```python
from build123d import *
from build123d.topology import SkipClean

# Parameters (mm, degrees)
SKETCH_1_R               = 30
EXTRUDE_1_DEPTH          = 8
CUT_EXTRUDE_5_DEPTH      = 905.685953271
CUT_EXTRUDE_5_DEPTH_BACK = 905.685953271
SKETCH_8_R               = 2.25
SKETCH_9_R               = 4
CUT_EXTRUDE_6_DEPTH      = 4.4
FILLET_1_R               = 100
CUT_EXTRUDE_7_DEPTH      = 83
CUT_EXTRUDE_8_DEPTH      = 83
FILLET_3_R               = 100
FILLET_4_R               = 10
SKETCH_14_R              = 4.25
CUT_EXTRUDE_9_DEPTH      = 83
EXTRUDE_2_DEPTH          = 5
CUT_EXTRUDE_10_DEPTH     = 69
FILLET_5_R               = 10
CHAMFER_1_SIZE           = 5
CHAMFER_2_SIZE           = 5


with BuildPart() as part:
    # 草图1 → 凸台-拉伸1 (new body)
    with BuildSketch(Plane.XY):
        Polygon((0, 250), (769.420884294, 0), (0, 0), (-100, 0), (-869.420884294, 0), (-100, 250), align=None)
        with Locations((100, 100)):
            Circle(SKETCH_1_R, mode=Mode.SUBTRACT)
        with Locations(Location((-200, 100, 0), (0, 0, 180))):
            Circle(SKETCH_1_R, mode=Mode.SUBTRACT)
    extrude(amount=EXTRUDE_1_DEPTH)

    # 草图8 → 切除-拉伸5 (cut, two sides: drawn at the far end of the back side and taken through both)
    with BuildSketch(Plane.XY.offset(8).offset(-CUT_EXTRUDE_5_DEPTH_BACK)):
        with Locations((100, 141.5)):
            Circle(SKETCH_8_R)
        with Locations((129.344931419, 129.344931419)):
            Circle(SKETCH_8_R)
        with Locations((141.5, 100)):
            Circle(SKETCH_8_R)
        with Locations((129.344931419, 70.655068581)):
            Circle(SKETCH_8_R)
        with Locations((100, 58.5)):
            Circle(SKETCH_8_R)
        with Locations((70.655068581, 70.655068581)):
            Circle(SKETCH_8_R)
        with Locations((58.5, 100)):
            Circle(SKETCH_8_R)
        with Locations((70.655068581, 129.344931419)):
            Circle(SKETCH_8_R)
        with Locations(Location((-170.655068581, 129.344931419, 0), (0, 0, 180))):
            Circle(SKETCH_8_R)
        with Locations(Location((-158.5, 100, 0), (0, 0, 180))):
            Circle(SKETCH_8_R)
        with Locations(Location((-170.655068581, 70.655068581, 0), (0, 0, 180))):
            Circle(SKETCH_8_R)
        with Locations(Location((-200, 58.5, 0), (0, 0, 180))):
            Circle(SKETCH_8_R)
        with Locations(Location((-229.344931419, 70.655068581, 0), (0, 0, 180))):
            Circle(SKETCH_8_R)
        with Locations(Location((-241.5, 100, 0), (0, 0, 180))):
            Circle(SKETCH_8_R)
        with Locations(Location((-229.344931419, 129.344931419, 0), (0, 0, 180))):
            Circle(SKETCH_8_R)
        with Locations(Location((-200, 141.5, 0), (0, 0, 180))):
            Circle(SKETCH_8_R)
    extrude(amount=CUT_EXTRUDE_5_DEPTH + CUT_EXTRUDE_5_DEPTH_BACK, mode=Mode.SUBTRACT)

    # 草图9 → 切除-拉伸6 (cut)
    with BuildSketch(Plane.XY.offset(8)):
        with Locations((-200, 141.5)):
            Circle(SKETCH_9_R)
        with Locations((-170.655068581, 129.344931419)):
            Circle(SKETCH_9_R)
        with Locations((-158.5, 100)):
            Circle(SKETCH_9_R)
        with Locations((-170.655068581, 70.655068581)):
            Circle(SKETCH_9_R)
        with Locations((-200, 58.5)):
            Circle(SKETCH_9_R)
        with Locations((-229.344931419, 70.655068581)):
            Circle(SKETCH_9_R)
        with Locations((-241.5, 100)):
            Circle(SKETCH_9_R)
        with Locations((-229.344931419, 129.344931419)):
            Circle(SKETCH_9_R)
        with Locations(Location((129.344931419, 129.344931419, 0), (0, 0, 180))):
            Circle(SKETCH_9_R)
        with Locations(Location((141.5, 100, 0), (0, 0, 180))):
            Circle(SKETCH_9_R)
        with Locations(Location((129.344931419, 70.655068581, 0), (0, 0, 180))):
            Circle(SKETCH_9_R)
        with Locations(Location((100, 58.5, 0), (0, 0, 180))):
            Circle(SKETCH_9_R)
        with Locations(Location((70.655068581, 70.655068581, 0), (0, 0, 180))):
            Circle(SKETCH_9_R)
        with Locations(Location((58.5, 100, 0), (0, 0, 180))):
            Circle(SKETCH_9_R)
        with Locations(Location((70.655068581, 129.344931419, 0), (0, 0, 180))):
            Circle(SKETCH_9_R)
        with Locations(Location((100, 141.5, 0), (0, 0, 180))):
            Circle(SKETCH_9_R)
    extrude(amount=-CUT_EXTRUDE_6_DEPTH, mode=Mode.SUBTRACT)

    # 圆角1
    fillet_1_edges = [part.edges().sort_by_distance(p)[0] for p in [
        (-869.420884294, 0, 4),
        (769.420884294, 0, 4),
    ]]
    fillet(fillet_1_edges, radius=FILLET_1_R)

    # 草图12 → 切除-拉伸7 (cut)
    with BuildSketch(Plane(origin=(0, 0, 0), x_dir=(-1, 0, 0), z_dir=(0, 0, -1))):
        with BuildLine():
            Line((-20, 40), (120, 40))
            ThreePointArc((120, 40), (155.27864045, 10.5572809), (200, 0))
            Line((200, 0), (-100, 0))
            ThreePointArc((-100, 0), (-55.27864045, 10.5572809), (-20, 40))
        make_face()
    extrude(amount=-CUT_EXTRUDE_7_DEPTH, mode=Mode.SUBTRACT)

    # 草图13 → 切除-拉伸8 (cut)
    with BuildSketch(Plane.XY.offset(8)):
        with BuildLine():
            Line((-238.045732826, 0), (-200, 0))
            ThreePointArc((-200, 0), (-295.54722537, 70.491904093), (-256.388333797, 182.585445519))
            Line((-256.388333797, 182.585445519), (-210, 214.258833414))
            Line((-210, 214.258833414), (-268.947432264, 195.10565163))
            ThreePointArc((-268.947432264, 195.10565163), (-336.814566886, 84.356553496), (-238.045732826, 0))
        make_face()
        with BuildLine():
            Line((110, 214.258833414), (168.947432264, 195.10565163))
            ThreePointArc((168.947432264, 195.10565163), (236.814566886, 84.356553496), (138.045732826, 0))
            Line((138.045732826, 0), (100, 0))
            ThreePointArc((100, 0), (195.54722537, 70.491904093), (156.388333797, 182.585445519))
            Line((156.388333797, 182.585445519), (110, 214.258833414))
        make_face()
    extrude(amount=-CUT_EXTRUDE_8_DEPTH, mode=Mode.SUBTRACT)

    # 圆角3
    fillet_3_edges = [part.edges().sort_by_distance(p)[0] for p in [
        (-100, 250, 4),
        (0, 250, 4),
        (-210, 214.258833414, 4),
        (110, 214.258833414, 4),
    ]]
    fillet(fillet_3_edges, radius=FILLET_3_R)

    # 圆角4
    fillet_4_edges = [part.edges().sort_by_distance(p)[0] for p in [
        (20, 40, 4),
        (-120, 40, 4),
    ]]
    fillet(fillet_4_edges, radius=FILLET_4_R)

    # 草图14 → 切除-拉伸9 (cut)
    with BuildSketch(Plane.XY.offset(8)):
        with Locations((-35, 65)):
            Circle(SKETCH_14_R)
        with Locations((-35, 105)):
            Circle(SKETCH_14_R)
        with Locations((-35, 175)):
            Circle(SKETCH_14_R)
        with Locations((-35, 215)):
            Circle(SKETCH_14_R)
        with Locations(Location((-65, 215, 0), (0, 0, 180))):
            Circle(SKETCH_14_R)
        with Locations(Location((-65, 175, 0), (0, 0, 180))):
            Circle(SKETCH_14_R)
        with Locations(Location((-65, 105, 0), (0, 0, 180))):
            Circle(SKETCH_14_R)
        with Locations(Location((-65, 65, 0), (0, 0, 180))):
            Circle(SKETCH_14_R)
    extrude(amount=-CUT_EXTRUDE_9_DEPTH, mode=Mode.SUBTRACT)

    # 草图15 → 凸台-拉伸2 (add)
    with SkipClean():  # the faces are left unmerged after this step: merging them gives an invalid solid
        with BuildSketch(Plane(origin=(0, 0, 0), x_dir=(-1, 0, 0), z_dir=(0, 0, -1))):
            with BuildLine():
                Line((-15.063255405, 245.10565163), (-96.358782137, 218.691133779))
                ThreePointArc((-96.358782137, 218.691133779), (-109.548764066, 213.340279426), (-121.845416496, 206.170927668))
                Line((-121.845416496, 206.170927668), (-156.388333797, 182.585445519))
                ThreePointArc((-156.388333797, 182.585445519), (-173.843422805, 32.567449192), (-22.861078416, 36.363636364))
                ThreePointArc((-22.861078416, 36.363636364), (-19.411200585, 39.045340337), (-15.147186258, 40))
                Line((-15.147186258, 40), (115.147186258, 40))
                ThreePointArc((115.147186258, 40), (119.411200585, 39.045340337), (122.861078416, 36.363636364))
                ThreePointArc((122.861078416, 36.363636364), (273.843422805, 32.567449192), (256.388333797, 182.585445519))
                Line((256.388333797, 182.585445519), (221.845416496, 206.170927668))
                ThreePointArc((221.845416496, 206.170927668), (209.548764066, 213.340279426), (196.358782137, 218.691133779))
                Line((196.358782137, 218.691133779), (115.063255405, 245.10565163))
                ThreePointArc((115.063255405, 245.10565163), (99.805002472, 248.76883406), (84.161555968, 250))
                Line((84.161555968, 250), (15.838444032, 250))
                ThreePointArc((15.838444032, 250), (0.194997528, 248.76883406), (-15.063255405, 245.10565163))
            make_face()
            with BuildLine():
                Line((55, 50), (128.192966918, 50))
                ThreePointArc((128.192966918, 50), (262.154722909, 38.412335488), (249.339792072, 172.262264829))
                Line((249.339792072, 172.262264829), (197.086815625, 207.939959117))
                Line((197.086815625, 207.939959117), (98.416155597, 240))
                Line((98.416155597, 240), (55, 240))
                Line((55, 240), (55, 50))
            make_face(mode=Mode.SUBTRACT)
            with BuildLine():
                Line((45, 240), (45, 50))
                Line((45, 50), (-28.192966918, 50))
                ThreePointArc((-28.192966918, 50), (-162.154722909, 38.412335488), (-149.339792072, 172.262264829))
                Line((-149.339792072, 172.262264829), (-97.086815625, 207.939959117))
                Line((-97.086815625, 207.939959117), (1.583844403, 240))
                Line((1.583844403, 240), (45, 240))
            make_face(mode=Mode.SUBTRACT)
        extrude(amount=EXTRUDE_2_DEPTH)

    # 草图16 → 切除-拉伸10 (cut)
    with SkipClean():  # the faces are left unmerged after this step: merging them gives an invalid solid
        with BuildSketch(Plane(origin=(0, 0, 0), x_dir=(-1, 0, 0), z_dir=(0, 0, -1))):
            Polygon((80, 230), (80, 130), (166.602540378, 180), align=None)
            Polygon((-66.602540378, 180), (20, 230), (20, 130), align=None)
        extrude(amount=-CUT_EXTRUDE_10_DEPTH, mode=Mode.SUBTRACT)

    # 圆角5
    fillet_5_edges = [part.edges().sort_by_distance(p)[0] for p in [
        (-197.086815625, 207.939959117, -2.5),
        (-98.416155597, 240, -2.5),
        (-55, 240, -2.5),
        (-55, 50, -2.5),
        (-128.192966918, 50, -2.5),
        (28.192966918, 50, -2.5),
        (-45, 50, -2.5),
        (-45, 240, -2.5),
        (-1.583844403, 240, -2.5),
        (97.086815625, 207.939959117, -2.5),
        (-80, 230, 4),
        (-166.602540378, 180, 4),
        (-80, 130, 4),
        (-20, 130, 4),
        (66.602540378, 180, 4),
        (-20, 230, 4),
    ]]
    fillet(fillet_5_edges, radius=FILLET_5_R)

    # 倒角1
    chamfer_1_edges = [part.edges().sort_by_distance(p)[0] for p in [
        (-273.843422805, 32.567449192, 8),
        (-239.116875146, 194.378186594, 8),
        (139.116875146, 194.378186594, 8),
        (-155.711018771, 231.898392704, 8),
        (55.711018771, 231.898392704, 8),
        (-50, 250, 8),
        (-209.548764066, 213.340279426, 8),
        (-99.805002472, 248.76883406, 8),
        (-0.194997528, 248.76883406, 8),
        (109.548764066, 213.340279426, 8),
        (173.843422805, 32.567449192, 8),
        (-50, 40, 8),
        (19.411200585, 39.045340337, 8),
        (-119.411200585, 39.045340337, 8),
        (-0.194997528, 248.76883406, -5),
        (55.711018771, 231.898392704, -5),
        (109.548764066, 213.340279426, -5),
        (139.116875146, 194.378186594, -5),
        (173.843422805, 32.567449192, -5),
        (19.411200585, 39.045340337, -5),
        (-50, 40, -5),
        (-119.411200585, 39.045340337, -5),
        (-273.843422805, 32.567449192, -5),
        (-239.116875146, 194.378186594, -5),
        (-209.548764066, 213.340279426, -5),
        (-155.711018771, 231.898392704, -5),
        (-99.805002472, 248.76883406, -5),
        (-50, 250, -5),
    ]]
    chamfer(chamfer_1_edges, length=CHAMFER_1_SIZE - 0.0001)  # a hair under: the kernel refuses the full size

    # 倒角2
    chamfer_2_edges = [part.edges().sort_by_distance(p)[0] for p in [
        (23.301270189, 155, 0),
        (23.301270189, 205, 0),
        (-20, 180, 0),
        (-123.301270189, 205, 0),
        (-123.301270189, 155, 0),
        (-80, 180, 0),
        (-156.602540378, 180, 0),
        (-85, 138.660254038, 0),
        (-85, 221.339745962, 0),
        (-15, 221.339745962, 0),
        (56.602540378, 180, 0),
        (-15, 138.660254038, 0),
    ]]
    chamfer(chamfer_2_edges, length=CHAMFER_2_SIZE)


solid = part.part
```
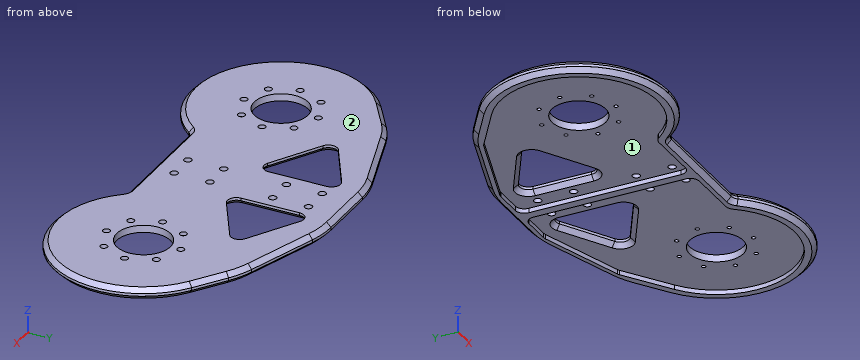
Check sheet for the modelled part. Datum: model origin and axes. Units: mm. Face numbers are marked on the shaded views. Coordinates: 2 decimals unless noted, no trailing zeros. Use a Markdown table: item, result.
1. Sectioned sample at A-A (z = -2.25). Give the number of separate pieces and of enclosed holes in the cut face, plus the area to 3 significant figures.
Reported:
| item | result |
|---|---|
| separate pieces | 1 |
| enclosed holes | 2 |
| area | 13,400 mm2 |
2. Release check for a two-part mould opening along X. For the marked faces 1 and 2 record: pulls with the +X half, pulls with the -X half, needs draft (parallel to the pull), parting line crosses it, or undercut.
Reported:
| item | result |
|---|---|
| face 1 | undercut |
| face 2 | needs draft |
3. Scan lines: line 1 along X through (y, z) = (139.5, 0.75); line 2 along X through (y, z) = (89.5, -2); line 3 along X through (y, z) = (190.5, -1.25). Record each from-to range of solid material in increasing order.
Reported:
| item | result |
|---|---|
| line 1 | x = -291.87 to -201.03, -198.97 to -104.95, -78.09 to -21.91, 4.95 to 98.97, 101.03 to 191.87 |
| line 2 | x = -297.44 to -286.87, -55 to -45, 186.87 to 197.44 |
| line 3 | x = -242.58 to -222.63, -55 to -45, 122.63 to 142.58 |
4. Go/stop test with flat-tipped pins: pin 1 Ø2 at (y, z) = (75.5, 1) entering from +X; pin 2 Ø2 at (x, z) = (62, 5.5) entering from +Y; pin 3 Ø6.5 at (x, y) = (100, 58.5) entering from -Z; pin 4 Ø11 at (x, y) = (-35, 105) entering from +Z. Record where each tip stops, or that it passes through.
Reported:
| item | result |
|---|---|
| pin 1 | stops at x = 197.2 |
| pin 2 | stops at y = 228.33 |
| pin 3 | stops at z = 0 |
| pin 4 | stops at z = 8 |
